Source: CAD feature listing. Evaluate the final solid. Frame: model axes, mm. A direction names the side the tool comes from. Give positions to 0.01 mm unless a question says otherwise; leave off trailing zeros. Write each loop counter-clockwise with the first axis right and the second up, starting at its lowest first coordinate (ties: lowest second). Pieces come first, ordered by that corner, then holes. Notation, with made-up numbers: (12, 63) - (51, 63) arc R12 ccw to (51, 81) - close; hole circle Ø7 at (45, 80.5). An arc over 180 degrees is marked (long way). One line per question, with ' | ' between items. Start each with the question number.
(1) Ray query, line 1 (Y direction, x = 0, z = 42.5); line 2 (Z direction, x = 2.5, y = 1); line 3 (Z direction, x = 7.5, y = 2). Return the intervals inside material, ascending. Write a range as [from, to].
(2) Pin query (flat end, axial travel): pin 1 (2 mm diameter, centred on x = 1.5, y = 0, fed in from -Z); pin 2 (1.5 mm diameter, centred on y = 3.5, z = 25, fed in from -X); pin 3 (2 mm diameter, centred on y = 2.5, z = 20, fed in from -X); pin 4 (6 mm diameter, centred on x = -1.5, z = 7.5, fed in from -Y). Return the tip coordinate at first contact, or that it passes through.
(3) Section C-C, the plane x = -5. Return loops of the section in (y, z), plus the area to 3 significant figures.
(4) Section A-A, the plane y = 0. Return loops of the section in (x, z), plus the area to 3 significant figures.
(5) Section B-B, the plane z = 32.5. Return loops of the section in (x, y), plus the area to 3 significant figures.
(6) Section D-D, the plane z = 16. Return loops of the section in (x, y).
(7) Draft query along Y for faces 3 (the flat face through (2, -6, 4)), 4 (the cylindrical face through (-6, 0, 28)), 5 (the flat face through (0, 0, 31)). Return one class per face: +Y half, -Y half, draft (parallel to the pull), parting line (faces both ways), or undercut.
(8) Access query for faces 1 (the cylindrical face through (-3, 0, 41)), 2 (the flat face through (0, 0, 0)). Directions: +Z, -Z, +X, -X, +Y, -Y. A direction counts if a zero-diameter tool reaches every point of the face in a straight line with its end or side. Return the directions, or none.
Autodesk Inventor part; units mm, degrees
ref_plane "YZ Plane" through (0, 0, 0) normal (1, 0, 0) x (0, 1, 0)
ref_plane "XZ Plane" through (0, 0, 0) normal (0, 1, 0) x (-1, 0, 0)
ref_plane "XY Plane" through (0, 0, 0) normal (0, 0, 1) x (1, 0, 0)
sketch "Sketch1" plane through (0, 0, 0) normal (0, 0, 1) x (1, 0, 0)
  circle A0 centre (0, 0) radius 9
  dimension "d0" = 18
extrude "Extrusion1" add sketch "Sketch1" along normal blind 4
sketch "Sketch2" plane through (0, 0, 4) normal (0, 0, 1) x (1, 0, 0)
  circle A0 centre (0, 0) radius 6
  circle A1 centre (0, 0) radius 3
  dimension "d3" = 12
  dimension "d4" = 6
extrude "Extrusion2" add sketch "Sketch2" along normal blind 48
sketch "Sketch4" plane through (0, 0, 4) normal (0, 0, 1) x (1, 0, 0)
  circle A0 centre (0, 0) radius 3
extrude "Extrusion3" add sketch "Sketch4" along normal blind 27
properties part number "Adaptateur_axes"
Check sheet entries:
1) line 1: [-6, -3], [3, 6] | line 2: [0, 31] | line 3: [0, 4]
2) pin 1: z = 0 | pin 2: x = -5.33 | pin 3: x = -5.81 | pin 4: y = -6
3) outline: (-7.48, 0) - (7.48, 0) - (7.48, 4) - (3.32, 4) - (3.32, 52) - (-3.32, 52) - (-3.32, 4) - (-7.48, 4) - close | area: 378 mm²
4) outline: (-9, 0) - (9, 0) - (9, 4) - (6, 4) - (6, 52) - (3, 52) - (3, 31) - (-3, 31) - (-3, 52) - (-6, 52) - (-6, 4) - (-9, 4) - close | area: 522 mm²
5) outline: circle Ø12 at (0, 0); hole circle Ø6 at (0, 0) | area: 84.8 mm²
6) outline: circle Ø12 at (0, 0)
7) face 3: draft | face 4: parting line | face 5: undercut
8) face 1: +Z | face 2: -Z, +X, -X, +Y, -Y
